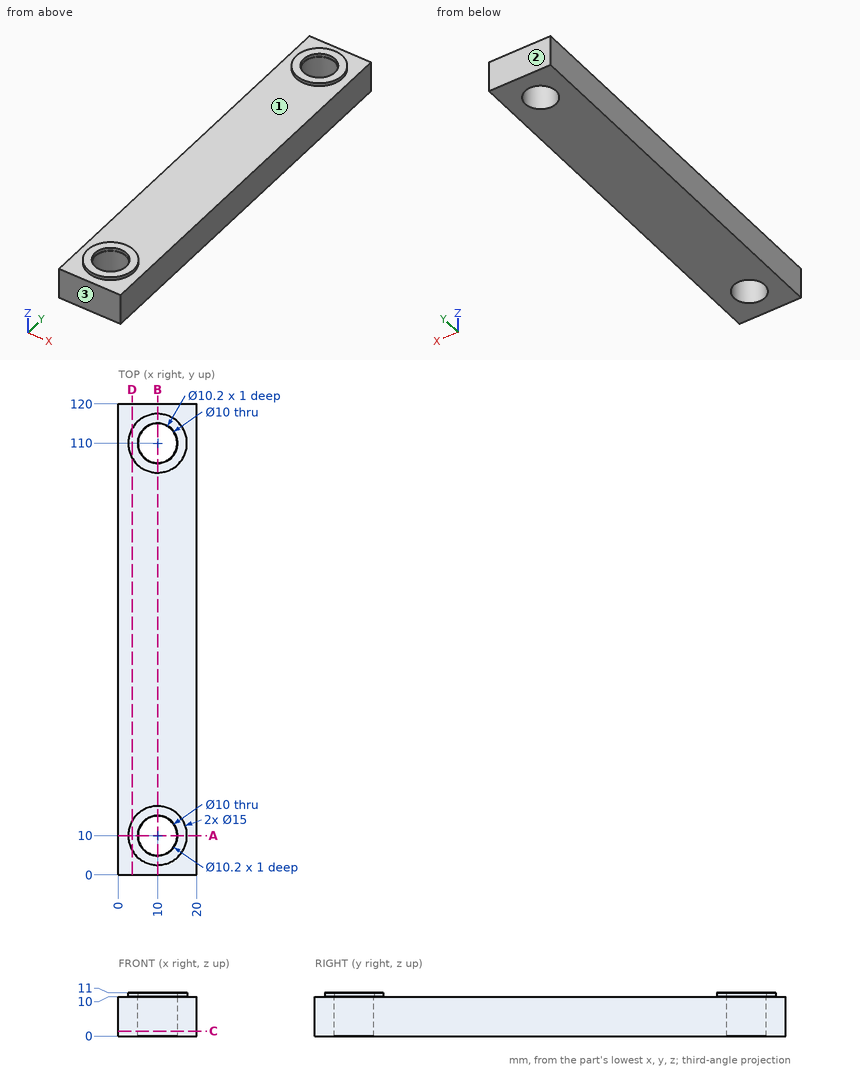
For this review, use the dimensioned drawing (mm, ordinates from the lowest corner) and the shaded views. Give positions to 0.01 mm unless a question says otherwise; leave off trailing zeros. Order: outer loops, then holes, each group sorted by start corner. A loop starts at its lowest first (then second) coordinate and runs counter-clockwise, first axis right, second up.
1) Insertion check: pin 1 (6 mm diameter, centred on x = 5, y = 86, fed in from +Z); pin 2 (6 mm diameter, centred on x = 10, y = 10, fed in from -Z). Each pin has a flat end and moves straight along its axis. Give the tip position at first contact, or say it passes through.
2) Take a section at B-B (x = 10). Give the boundary of the cut face in (y, z), then the cut area to 3 significant figures.
3) Take a section at C-C (z = 1.25). Give the boundary of the cut face in (x, y), then the cut area to 3 significant figures.
4) The part is to be moulded in two halves that separate along Y. For the marked faces 1, 2 and 3, say which applies: released by +Y, released by -Y, zero draft, split by the parting line, or undercut.
5) Take a section at A-A (y = 10). Give the boundary of the cut face in (x, z).
6) Take a section at D-D (x = 3.5). Give the boundary of the cut face in (y, z), then the cut area to 3 significant figures.
7) Wall thickness on line 1 (Y direction, x = 10, z = 5); line 2 (Y direction, x = 10, z = 10.7); line 3 (Y direction, x = 8.5, z = 2.75): over which ranges is each line inside the solid? List them lowest first.
Derived:
1. pin 1: stops at z = 10
1. pin 2: passes through
2. outline: (0, 0) - (5, 0) - (5, 10) - (4.9, 10) - (4.9, 11) - (2.5, 11) - (2.5, 10) - (0, 10) - close; (15, 0) - (105, 0) - (105, 10) - (104.9, 10) - (104.9, 11) - (102.5, 11) - (102.5, 10) - (17.5, 10) - (17.5, 11) - (15.1, 11) - (15.1, 10) - (15, 10) - close; (115, 0) - (120, 0) - (120, 10) - (117.5, 10) - (117.5, 11) - (115.1, 11) - (115.1, 10) - (115, 10) - close
2. area: 1,010 mm2
3. outline: (0, 0) - (20, 0) - (20, 120) - (0, 120) - close; hole circle Ø10 at (10, 10); hole circle Ø10 at (10, 110)
3. area: 2,240 mm2
4. face 1: undercut
4. face 2: released by +Y
4. face 3: released by -Y
5. outline: (0, 0) - (5, 0) - (5, 10) - (4.9, 10) - (4.9, 11) - (2.5, 11) - (2.5, 10) - (0, 10) - close; (15, 0) - (20, 0) - (20, 10) - (17.5, 10) - (17.5, 11) - (15.1, 11) - (15.1, 10) - (15, 10) - close
6. outline: (0, 0) - (120, 0) - (120, 10) - (113.74, 10) - (113.74, 11) - (106.26, 11) - (106.26, 10) - (13.74, 10) - (13.74, 11) - (6.26, 11) - (6.26, 10) - (0, 10) - close
6. area: 1,210 mm2
7. line 1: y = 0 to 5, 15 to 105, 115 to 120
7. line 2: y = 2.5 to 4.9, 15.1 to 17.5, 102.5 to 104.9, 115.1 to 117.5
7. line 3: y = 0 to 5.23, 14.77 to 105.23, 114.77 to 120
